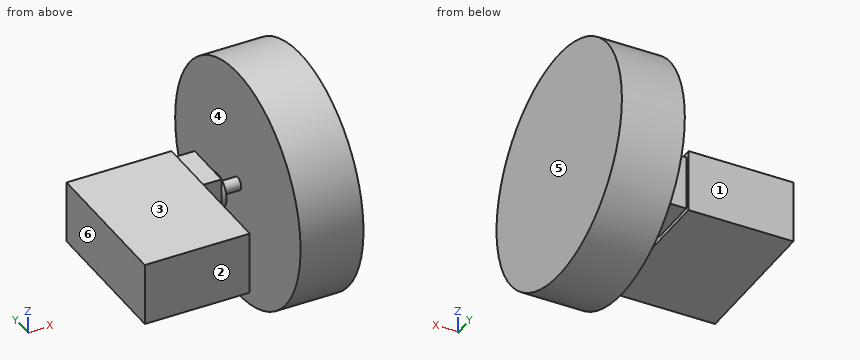
```python
from build123d import *

# Parameters (mm, degrees)
SKETCH_1_W           = 25
SKETCH_1_H           = 35
EXTRUDE_1_DEPTH      = 15
SKETCH_3_W           = 13
SKETCH_3_H           = 12
EXTRUDE_2_DEPTH      = 5
EXTRUDE_START        = 30
SKETCH_4_R           = 4
EXTRUDE_3_DEPTH      = 2
EXTRUDE_4_DEPTH      = 4.819582841
EXTRUDE_4_DEPTH_BACK = 2
EXTRUDE_4_START      = 32
SKETCH_5_R           = 1.5
EXTRUDE_START_2      = 36.819583
SKETCH_6_R           = 28.053339705
EXTRUDE_5_DEPTH      = 15


with BuildPart() as part:
    # 草图1 → 凸台-拉伸1 (new body)
    with BuildSketch(Plane.XY):
        with Locations((12.5, -17.5)):
            Rectangle(SKETCH_1_W, SKETCH_1_H)
    extrude(amount=EXTRUDE_1_DEPTH)

    # 草图3 → 凸台-拉伸2 (add)
    with BuildSketch(Plane(origin=(25, 0, 0), x_dir=(0, 0, -1), z_dir=(1, 0, 0))):
        with Locations((-7.5, -7)):
            Rectangle(SKETCH_3_W, SKETCH_3_H)
    extrude(amount=EXTRUDE_2_DEPTH)

    # 草图4 → 凸台-拉伸3 (add)
    with BuildSketch(Plane(origin=(0, 0, 0), x_dir=(0, 0, -1), z_dir=(1, 0, 0)).offset(EXTRUDE_START)):
        with Locations(Location((-7.5, -7.5, 0), (0, 0, 90))):
            Circle(SKETCH_4_R)
    extrude(amount=EXTRUDE_3_DEPTH)

    # 草图5 → 凸台-拉伸4 (add, two sides: drawn at the far end of the back side and taken through both)
    with BuildSketch(Plane(origin=(0, 0, 0), x_dir=(0, 0, -1), z_dir=(1, 0, 0)).offset(EXTRUDE_4_START - EXTRUDE_4_DEPTH_BACK)):
        with Locations(Location((-7.5, -7.5, 0), (0, 0, 90))):
            Circle(SKETCH_5_R)
    extrude(amount=EXTRUDE_4_DEPTH + EXTRUDE_4_DEPTH_BACK)

    # 草图6 → 凸台-拉伸5 (add)
    with BuildSketch(Plane(origin=(0, 0, 0), x_dir=(0, 0, -1), z_dir=(1, 0, 0)).offset(EXTRUDE_START_2)):
        with Locations(Location((-7.5, -7.5, 0), (0, 0, 90))):
            Circle(SKETCH_6_R)
    extrude(amount=EXTRUDE_5_DEPTH)


solid = part.part
```
Geometry: final body of the model. Coordinates: model frame, mm. Face numbers are marked on the shaded views. A direction names the side the tool comes from. Coordinates: 2 decimals unless noted, no trailing zeros. Write each loop counter-clockwise with the first axis right and the second up, starting at its lowest first coordinate (ties: lowest second). Pieces come first, ordered by that corner, then holes. Notation, with made-up numbers: M 89,33 L 107,33 A30 ccw 107,61 Z; hole C 8.5,-34 d2. An arc over 180 degrees is marked long. Use CSV: the item, a comma, the result in double quotes. Start each with the question number.
1. Mould query, pull axis X, two halves, no side actions, for the marked faces 4, 5 and 6. Classes: pulls with the +X half, pulls with the -X half, needs draft (parallel to the pull), parting line crosses it, or undercut.
2. First-contact query: P1, Ø8, axis at x = 35, z = -11, coming from the -Y side; P2, Ø1.5, axis at x = 13, z = 12.5, coming from the +Y side; P3, Ø1.5, axis at y = 14, z = -6.5, coming from the -X side; P4, Ø10, axis at y = 12.5, z = -14, coming from the +X side. Flat tips, straight axial feed; report the tip coordinate or a pass-through.
3. Cut plane C-C on y = -7.5. Return the cut outline in (x, z).
4. Cut plane A-A on y = -23.5. Return the cut outline in (x, z).
5. Cut plane D-D on x = 6.5. Return the cut outline in (y, z), plus the area to 3 significant figures.
6. Reachability of the marked faces 1, 2 and 3 from +Z, -Z, +X, -X, +Y, -Y: full face, straight path, thin tool, end or side. Return the list, or none.
7. Ray query, probe 1 along X at (y, z) = (-30, 11.5); probe 2 along X at (y, z) = (-1, -16); probe 3 along Y at (x, z) = (9.5, 3.5). Return the intervals inside material, ascending.
8. Cut plane B-B on z = 7.5. Return the cut outline in (x, y), plus the area to 3 significant figures.
Entries:
1,face 4,"undercut"
1,face 5,"pulls with the +X half"
1,face 6,"pulls with the -X half"
2,P1,"y = -31.25"
2,P2,"y = 0"
2,P3,"x = 36.82"
2,P4,"x = 51.82"
3,outline,"M 0,0 L 25,0 L 25,1 L 30,1 L 30,3.5 L 32,3.5 L 32,6 L 36.82,6 L 36.82,-20.55 L 51.82,-20.55 L 51.82,35.55 L 36.82,35.55 L 36.82,9 L 32,9 L 32,11.5 L 30,11.5 L 30,14 L 25,14 L 25,15 L 0,15 Z"
4,outline,"M 0,0 L 25,0 L 25,15 L 0,15 Z; M 36.82,-15.54 L 51.82,-15.54 L 51.82,30.54 L 36.82,30.54 Z"
5,outline,"M -35,0 L 0,0 L 0,15 L -35,15 Z"
5,area,"525 mm²"
6,face 1,"+Z, -Z, -X, +Y"
6,face 2,"+Z, -Z, -X, -Y"
6,face 3,"+Z, -X, +Y, -Y"
7,probe 1,"0 to 25, 36.82 to 51.82"
7,probe 2,"36.82 to 51.82"
7,probe 3,"-35 to 0"
8,outline,"M 0,-35 L 25,-35 L 25,-13 L 30,-13 L 30,-11.5 L 32,-11.5 L 32,-9 L 36.82,-9 L 36.82,-35.55 L 51.82,-35.55 L 51.82,20.55 L 36.82,20.55 L 36.82,-6 L 32,-6 L 32,-3.5 L 30,-3.5 L 30,-1 L 25,-1 L 25,0 L 0,0 Z"
8,area,"1,810 mm²"
